from build123d import *

# Parameters (mm, degrees)
F1_DEPTH = 5
F0_W     = 34.5
F0_H     = 52.5
F2_DEPTH = 8.4
F0_W_2   = 3.25
F0_H_2   = 19
F0_W_3   = 19
F0_H_3   = 3.25
F3_DEPTH = 9.5


with BuildPart() as f1:
    # F0 (on Front) → F1 (new body)
    with BuildSketch(Plane.XZ):
        Polygon((-3.162847, 112.5443), (-26.912847, 112.5443), (-26.912847, 67.5443), (-26.912847, 48.5443), (-18.662847, 48.5443), (-18.662847, 101.0443), (15.837153, 101.0443), (15.837153, 112.5443), align=None)
        Polygon((34.837153, 112.5443), (15.837153, 112.5443), (15.837153, 101.0443), (50.337153, 101.0443), (50.337153, 48.5443), (58.587153, 48.5443), (58.587153, 67.5443), (58.587153, 112.5443), align=None)
        Polygon((58.587153, 48.5443), (50.337153, 48.5443), (50.337153, -3.9557), (15.837153, -3.9557), (15.837153, -15.4557), (34.837153, -15.4557), (58.587153, -15.4557), (58.587153, 29.5443), align=None)
        Polygon((-18.662847, 48.5443), (-26.912847, 48.5443), (-26.912847, 29.5443), (-26.912847, -15.4557), (-3.162847, -15.4557), (15.837153, -15.4557), (15.837153, -3.9557), (-18.662847, -3.9557), align=None)
    extrude(amount=F1_DEPTH)

    # F0 (on Front) → F2 (join)
    with BuildSketch(Plane.XZ):
        with Locations((-1.412847, 74.7943)):
            Rectangle(F0_W, F0_H)
        with Locations((33.087153, 74.7943)):
            Rectangle(F0_W, F0_H)
        with Locations((33.087153, 22.2943)):
            Rectangle(F0_W, F0_H)
        with Locations((-1.412847, 22.2943)):
            Rectangle(F0_W, F0_H)
    extrude(amount=F2_DEPTH)

    # F0 (on Front) → F3 (join)
    with BuildSketch(Plane.XZ):
        with Locations((-28.537847, 58.0443)):
            Rectangle(F0_W_2, F0_H_2)
        with Locations((-28.537847, 39.0443)):
            Rectangle(F0_W_2, F0_H_2)
        with Locations((6.337153, 114.1693)):
            Rectangle(F0_W_3, F0_H_3)
        with Locations((25.337153, 114.1693)):
            Rectangle(F0_W_3, F0_H_3)
        with Locations((60.212153, 58.0443)):
            Rectangle(F0_W_2, F0_H_2)
        with Locations((60.212153, 39.0443)):
            Rectangle(F0_W_2, F0_H_2)
        with Locations((25.337153, -17.0807)):
            Rectangle(F0_W_3, F0_H_3)
        with Locations((6.337153, -17.0807)):
            Rectangle(F0_W_3, F0_H_3)
    extrude(amount=F3_DEPTH)


solid = f1.part
Source: CAD feature listing. Evaluate the final solid. Frame: model axes, mm. A direction names the side the tool comes from. Give positions to 0.01 mm unless a question says otherwise; leave off trailing zeros. Order: outer loops, then holes, each group sorted by start corner. A loop starts at its lowest first (then second) coordinate and runs counter-clockwise, first axis right, second up. Notation, with made-up numbers: (75.5, 36) -> (115.5, 36) arc R21 cw to (115.5, 69) -> close; hole circle Ø11 at (35, 56). An arc over 180 degrees is marked (long way). Write item = value, one per line.
Q1. Cut plane B-B, the plane x = 2. Output: boundary loops of the cut face in (y, z).
Data:
outline = (-9.5, -18.71) -> (0, -18.71) -> (0, 115.79) -> (-9.5, 115.79) -> (-9.5, 112.54) -> (-5, 112.54) -> (-5, 101.04) -> (-8.4, 101.04) -> (-8.4, -3.96) -> (-5, -3.96) -> (-5, -15.46) -> (-9.5, -15.46) -> close
Q2. Cut plane D-D, the plane z = 36. Output: boundary loops of the cut face in (x, y), and give its area (3 significant figures).
Data:
outline = (-30.16, -9.5) -> (-26.91, -9.5) -> (-26.91, -5) -> (-18.66, -5) -> (-18.66, -8.4) -> (50.34, -8.4) -> (50.34, -5) -> (58.59, -5) -> (58.59, -9.5) -> (61.84, -9.5) -> (61.84, 0) -> (-30.16, 0) -> close
area = 724 mm^2
Q3. Pull-direction query (Z, two-part tool) for faces 1 (the face through (16, -9.5, -17)), 2 (the face through (60, -5, 29.544)), 3 (the face through (53, -5, 49)); classes: released by +Z, released by -Z, zero draft, split by the parting line, or undercut.
Data:
face_1 = zero draft
face_2 = released by -Z
face_3 = undercut
Q4. Cut plane A-A, the plane y = -7. Output: boundary loops of the cut face in (x, z).
Data:
outline = (-30.16, 29.54) -> (-26.91, 29.54) -> (-26.91, 67.54) -> (-30.16, 67.54) -> close; (-18.66, -3.96) -> (50.34, -3.96) -> (50.34, 101.04) -> (-18.66, 101.04) -> close; (-3.16, -18.71) -> (34.84, -18.71) -> (34.84, -15.46) -> (-3.16, -15.46) -> close; (-3.16, 112.54) -> (34.84, 112.54) -> (34.84, 115.79) -> (-3.16, 115.79) -> close; (58.59, 29.54) -> (61.84, 29.54) -> (61.84, 67.54) -> (58.59, 67.54) -> close
Q5. Cut plane C-C, the plane z = 99.5. Output: boundary loops of the cut face in (x, y), and give its area (3 significant figures).
Data:
outline = (-26.91, -5) -> (-18.66, -5) -> (-18.66, -8.4) -> (50.34, -8.4) -> (50.34, -5) -> (58.59, -5) -> (58.59, 0) -> (-26.91, 0) -> close
area = 662 mm^2
Q6. Set-up query: faces 4 (the face through (-26.913, -2, 90)), 5 (the face through (16, -7, 112.544)), 6 (the face through (34.837, -5, -17)), 7 (the face through (-3.163, -5, -17)). Return all of +Z, -Z, +X, -X, +Y, -Y with unobstructed straight access to the full face (end or side cutting, diameter ignored); none if empty.
Data:
face_4 = +Z, -X, +Y, -Y
face_5 = +X, -X, -Y
face_6 = -Z, +X, +Y, -Y
face_7 = -Z, -X, +Y, -Y
Q7. Material intervals for line 1 (Z direction, x = 24.5, y = -5.75); line 2 (Z direction, x = 22, y = -8.5); line 3 (Y direction, x = 47.5, z = 20), sorted ascending. Write a range as from..to.
Data:
line_1 = -18.71..-15.46, -3.96..101.04, 112.54..115.79
line_2 = -18.71..-15.46, 112.54..115.79
line_3 = -8.4..0
Q8. Pin query (flat end, axial travel): pin 1 (2.5 mm diameter, centred on y = -3, z = 85, fed in from +X); pin 2 (12 mm diameter, centred on x = 1, z = 11, fed in from -Y); pin 3 (2.5 mm diameter, centred on y = -5.5, z = -17, fed in from +X). Return the tip coordinate at first contact, or that it passes through.
Data:
pin_1 = 58.59
pin_2 = -8.4
pin_3 = 34.84
